```python
from build123d import *

# Parameters (mm, degrees)
CHAMFER1_SIZE         = 1
CUT_EXTRUDE1_DEPTH    = 4
CUT_EXTRUDE2_DEPTH    = 10
M8_TAPPED_HOLE1_D     = 6.8
M8_TAPPED_HOLE1_DEPTH = 19.75
M8_TAPPED_HOLE1_TIP   = 2.042926105
CHAMFER2_SIZE         = 1


with BuildPart() as part:
    # Sketch1 → Revolve1 (revolve)
    with BuildSketch(Plane.XY, mode=Mode.PRIVATE) as revolve1_sk:
        Polygon((0, 0), (0, 12.5), (38.6, 12.5), (38.6, 15), (43.6, 15), (43.6, 12), (44.6, 12), (44.6, 12.5), (120.2, 12.5), (120.2, 0), align=None)
    revolve(revolve1_sk.sketch.rotate(Axis((0, 0, 0), (-1, 0, 0)), 90), axis=Axis((0, 0, 0), (-1, 0, 0)))

    # Chamfer1
    chamfer1_edges = [part.edges().sort_by_distance(p)[0] for p in [
        (0, 0, 12.5),
    ]]
    chamfer(chamfer1_edges, length=CHAMFER1_SIZE)

    # Sketch3 → Cut-Extrude1 (cut)
    with BuildSketch(Plane(origin=(120.2, 2.936266506, 12.5), x_dir=(1, 0, 0), z_dir=(0, 0, -1))):
        with BuildLine():
            Line((-5, 6.936266506), (-50, 6.936266506))
            ThreePointArc((-50, 6.936266506), (-54, 2.936266506), (-50, -1.063733494))
            Line((-50, -1.063733494), (-5, -1.063733494))
            ThreePointArc((-5, -1.063733494), (-1, 2.936266506), (-5, 6.936266506))
        make_face()
    extrude(amount=CUT_EXTRUDE1_DEPTH, mode=Mode.SUBTRACT)

    # Sketch4 → Cut-Extrude2 (cut)
    with BuildSketch(Plane(origin=(120.2, 0, 0), x_dir=(0, 0, -1), z_dir=(1, 0, 0))):
        with BuildLine():
            Line((-8.5, -4), (-8.5, 4))
            Line((-8.5, 4), (-11.842719282, 4))
            ThreePointArc((-11.842719282, 4), (-12.5, 0), (-11.842719282, -4))
            Line((-11.842719282, -4), (-8.5, -4))
        make_face()
    extrude(amount=-CUT_EXTRUDE2_DEPTH, mode=Mode.SUBTRACT)

    # M8 Tapped Hole1
    with Locations(Plane(origin=(120.2, 0, 0), x_dir=(0, 0, -1), z_dir=(1, 0, 0))):
        with Locations((0, 0)):
            Hole(M8_TAPPED_HOLE1_D / 2, depth=M8_TAPPED_HOLE1_DEPTH)
            with Locations((0, 0, -(M8_TAPPED_HOLE1_DEPTH + M8_TAPPED_HOLE1_TIP / 2))):  # 118° drill point
                Cone(0, M8_TAPPED_HOLE1_D / 2, M8_TAPPED_HOLE1_TIP, mode=Mode.SUBTRACT)

    # Chamfer2
    chamfer2_edges = [part.edges().sort_by_distance(p)[0] for p in [
        (120.2, 12.33458534, -2.026821276),
    ]]
    chamfer(chamfer2_edges, length=CHAMFER2_SIZE)


solid = part.part
```
Input: part model. Units: mm. Frame: model coordinates. A direction names the side the tool comes from. Give positions to 0.01 mm unless a question says otherwise; leave off trailing zeros. Loops run counter-clockwise (first coordinate to the right, second up) from the corner with the lowest first, then second, coordinate; pieces in that order, holes last.
1) Section query B-B on x = 90. Return the cut outline in (y, z), and give its area (3 significant figures).
A:
outline: (-4, 8.5) - (-4, 11.84) arc R12.5 ccw (long way) to (4, 11.84) - (4, 8.5) - close
area: 461 mm2
2) Contact query for flat-ended pins moving along their axis: pin 1 (10 mm diameter, centred on x = 34.5, z = 0, fed in from -Y); pin 2 (4 mm diameter, centred on y = 0, z = 0, fed in from +X); pin 3 (12 mm diameter, centred on x = 42, y = 8.5, fed in from +Z); pin 4 (1 mm diameter, centred on x = 97.5, z = 10, fed in from -Y). Output: stop coordinate, or through.
A:
pin 1: stops at y = -15
pin 2: stops at x = 99.61
pin 3: stops at z = 14.79
pin 4: stops at y = -8.12
3) Line query: L1, parallel to Y at x = 107.75, z = 0; L2, parallel to X at y = -7.75, z = 11.5; L3, parallel to Y at x = 51.5, z = 0. Output: solid intervals per line, ascending.
A:
L1: y = -12.5 to -3.4, 3.4 to 12.5
L2: x = 38.6 to 43.6
L3: y = -12.5 to 12.5
4) Reachability of faces 4 (the cylindrical face through (82.422, -3.755, -11.923)), 5 (the flat face through (94, 0, 8.5)), 6 (the flat face through (44.6, -10, -7)) from +Z, -Z, +X, -X, +Y, -Y: full face, straight path, thin tool, end or side. Return the list, or none.
A:
face 4: +X
face 5: +Z, +X
face 6: none
5) Section query A-A on x = 52. Return the cut outline in (y, z).
A:
outline: circle Ø25 at (0, 0)
6) Mould query, pull axis Y, two halves, no side actions, for faces 1 (the cylindrical face through (66.2, -0.1, 10.5)), 2 (the cylindrical face through (20.063, -3.755, -11.923)), 3 (the flat face through (38.6, -12.3, -3.4)). Classes: released by +Y, released by -Y, zero draft, split by the parting line, or undercut.
A:
face 1: undercut
face 2: split by the parting line
face 3: zero draft
